The model under review builds one solid part; all positions refer to its coordinate system, in mm. Coordinates: 2 decimals unless noted, no trailing zeros. Write each loop counter-clockwise with the first axis right and the second up, starting at its lowest first coordinate (ties: lowest second). Pieces come first, ordered by that corner, then holes. Notation, with made-up numbers: (-17, -4.5) - (16, -4.5) arc R21 cw to (16, 26.5) - close; hole circle Ø7 at (10, 47.25). An arc over 180 degrees is marked (long way). Use one line per item in the form item = value. Start each with the question number.
Autodesk Inventor part; units mm, degrees
ref_plane "YZ Plane" through (0, 0, 0) normal (1, 0, 0) x (0, 1, 0)
ref_plane "XZ Plane" through (0, 0, 0) normal (0, 1, 0) x (-1, 0, 0)
ref_plane "XY Plane" through (0, 0, 0) normal (0, 0, 1) x (1, 0, 0)
sketch "Sketch1" plane through (0, 0, 0) normal (0, 1, 0) x (-1, 0, 0)
  line L0 (70, 0) -> (-70, 0) construction
  line L1 (0, -70) -> (0, 70) construction
  line L2 (-50, 50) -> (50, 50)
  line L3 (50, 50) -> (50, -50)
  line L4 (50, -50) -> (-50, -50)
  line L5 (-50, -50) -> (-50, 50)
  line L6 (-50, 50) -> (50, -50) construction
  line L7 (50, 50) -> (-50, -50) construction
  circle A0 centre (0, 0) radius 5
  dimension "d0" = 100
  dimension "d3" = 10
extrude "Extrusion1" add sketch "Sketch1" along normal blind 12
properties part number "Manual_NC_REF"
1. The part is to be moulded in two halves that separate along Z. For faces 1 (the cylindrical face through (1.08, 5.92, 4.88)), 2 (the flat face through (-1, 6, -50)), 3 (the flat face through (-50, 6, 1)), say which applies: released by +Z, released by -Z, zero draft, split by the parting line, or undercut.
2. For P1, Ø8, axis at x = 0, z = 0, coming from the +Y side, flat-tipped, find the tip position at first contact; note if it passes through.
3. Take a section at B-B (z = 0). State the section outline as (x, y) points.
4. Take a section at A-A (x = 0). State the section outline as (y, z) points, plus the area to 3 significant figures.
5. For L1, parallel to Z at x = 0, y = 8.75; L2, parallel to Z at x = -3.5, y = 8.25, list the stretches that pass through material, from the lowest coordinate up.
Returned:
q1.face_1 = undercut
q1.face_2 = released by -Z
q1.face_3 = zero draft
q2.P1 = through
q3.outline = (-50, 0) - (-5, 0) - (-5, 12) - (-50, 12) - close; (5, 0) - (50, 0) - (50, 12) - (5, 12) - close
q4.outline = (0, -50) - (12, -50) - (12, -5) - (0, -5) - close; (0, 5) - (12, 5) - (12, 50) - (0, 50) - close
q4.area = 1,080 mm²
q5.L1 = -50 to -5, 5 to 50
q5.L2 = -50 to -3.57, 3.57 to 50
